Design review of the part built by this model. Coordinates are the model's own, in mm. Face numbers are marked on the shaded views. A direction names the side the tool comes from. Round coordinates to 2 decimals unless told otherwise and drop trailing zeros. Write each loop counter-clockwise with the first axis right and the second up, starting at its lowest first coordinate (ties: lowest second). Pieces come first, ordered by that corner, then holes. Notation, with made-up numbers: (21, 9.5) -> (45, 9.5) arc R21 cw to (45, 35.5) -> close; hole circle Ø11 at (-18, 38). An arc over 180 degrees is marked (long way). One line per question, with ' | ' between items. Start each with the question number.
1) Insertion check: pin 1 Ø0.9 at (x, y) = (-105.5, -7.5) entering from -Z; pin 2 Ø5 at (x, y) = (-97.5, 8.5) entering from +Z. Each pin has a flat end and moves straight along its axis. Give the tip position at first contact, or say it passes through.
2) Consider section A-A (z = 14.5). Give the boundary of the cut face in (x, y).
3) For the marked faces 1 and 2, list the 3-axis set-ups (+Z, -Z, +X, -X, +Y, -Y) from which the entire face can be reached by the end or side of a thin tool; tool diameter is ignored.
4) Consider section D-D (z = 6). Give the boundary of the cut face in (x, y), then the cut area to 3 significant figures.
5) Mouldability with a two-part tool opening along X and no side actions: class the marked faces 3, 4, 5 and 6 as +X half, -X half, draft (parallel to the pull), parting line (faces both ways), or undercut.
6) Consider section B-B (x = -92). Give the boundary of the cut face in (y, z), then the cut area to 3 significant figures.
7) For probe 1 along X at (y, z) = (1, 13.75); probe 2 along Y at (x, z) = (-91, 10.5); probe 3 along Z at (x, y) = (-87, -3.5), list the stretches that pass through material, from the lowest coordinate up.
8) Consider section C-C (y = 3). Give the boundary of the cut face in (x, z).
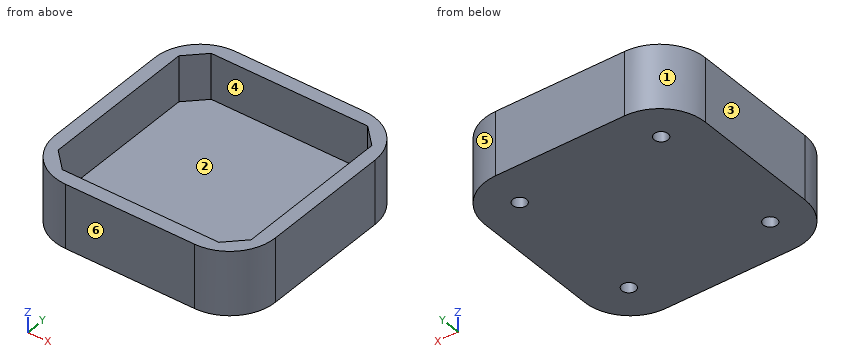
```python
from build123d import *

# Parameters (mm, degrees)
SKETCH1_W           = 48.3
SKETCH1_H           = 48.3
BOSS_EXTRUDE1_DEPTH = 10
SKETCH1_3_W         = 48.3
SKETCH1_3_H         = 48.3
SKETCH1_3_R         = 3.6
SKETCH1_3_R_2       = 6.5
BOSS_EXTRUDE2_DEPTH = 4
SKETCH2_R           = 1.5
CUT_EXTRUDE1_DEPTH  = 3.5
FILLET1_R           = 10


with BuildPart() as part:
    # Sketch1 → Boss-Extrude1 (new body)
    with BuildSketch(Plane(origin=(0, 0, 7.613932461), x_dir=(-1, 0, 0), z_dir=(0, 0, -1))):
        with Locations((89.733633233, 8.444815184)):
            Rectangle(SKETCH1_W, SKETCH1_H)
        Polygon((72.583633233, 29.594815184), (68.583633233, 25.594815184), (68.583633233, -8.705184816), (72.583633233, -12.705184816), (106.883633233, -12.705184816), (110.883633233, -8.705184816), (110.883633233, 25.594815184), (106.883633233, 29.594815184), align=None, mode=Mode.SUBTRACT)
    extrude(amount=-BOSS_EXTRUDE1_DEPTH)

    # Sketch1_3 → Boss-Extrude2 (add)
    with BuildSketch(Plane(origin=(0, 0, 7.613932461), x_dir=(-1, 0, 0), z_dir=(0, 0, -1))):
        with Locations((89.733633233, 8.444815184)):
            Rectangle(SKETCH1_3_W, SKETCH1_3_H)
        Polygon((72.583633233, 29.594815184), (68.583633233, 25.594815184), (68.583633233, -8.705184816), (72.583633233, -12.705184816), (106.883633233, -12.705184816), (110.883633233, -8.705184816), (110.883633233, 25.594815184), (106.883633233, 29.594815184), align=None, mode=Mode.SUBTRACT)
        Polygon((106.883633233, 29.594815184), (72.583633233, 29.594815184), (68.583633233, 25.594815184), (68.583633233, -8.705184816), (72.583633233, -12.705184816), (106.883633233, -12.705184816), (110.883633233, -8.705184816), (110.883633233, 25.594815184), align=None)
        Polygon((106.46941967, -11.705184816), (109.883633233, -8.290971253), (109.883633233, 25.180601622), (106.46941967, 28.594815184), (72.997846795, 28.594815184), (69.583633233, 25.180601622), (69.583633233, -8.290971253), (72.997846795, -11.705184816), align=None, mode=Mode.SUBTRACT)
        Polygon((72.997846795, -11.705184816), (106.46941967, -11.705184816), (109.883633233, -8.290971253), (109.883633233, 25.180601622), (106.46941967, 28.594815184), (72.997846795, 28.594815184), (69.583633233, 25.180601622), (69.583633233, -8.290971253), align=None)
        with Locations((105.233633233, -7.055184816)):
            Circle(SKETCH1_3_R, mode=Mode.SUBTRACT)
        with Locations((74.233633233, 23.944815184)):
            Circle(SKETCH1_3_R, mode=Mode.SUBTRACT)
        with Locations((89.733633233, 8.444815184)):
            Circle(SKETCH1_3_R_2, mode=Mode.SUBTRACT)
        with Locations((105.233633233, 23.944815184)):
            Circle(SKETCH1_3_R, mode=Mode.SUBTRACT)
        with Locations((74.233633233, -7.055184816)):
            Circle(SKETCH1_3_R, mode=Mode.SUBTRACT)
        with Locations((105.233633233, 23.944815184)):
            Circle(SKETCH1_3_R)
        with Locations((89.733633233, 8.444815184)):
            Circle(SKETCH1_3_R_2)
        with Locations((105.233633233, -7.055184816)):
            Circle(SKETCH1_3_R)
        with Locations((74.233633233, -7.055184816)):
            Circle(SKETCH1_3_R)
        with Locations((74.233633233, 23.944815184)):
            Circle(SKETCH1_3_R)
    extrude(amount=BOSS_EXTRUDE2_DEPTH)

    # Sketch2 → Cut-Extrude1 (cut)
    with BuildSketch(Plane(origin=(0, 0, 3.613932461), x_dir=(-1, 0, 0), z_dir=(0, 0, -1))):
        with Locations((105.233633233, 23.944815184)):
            Circle(SKETCH2_R)
        with Locations((105.233633233, -7.055184816)):
            Circle(SKETCH2_R)
        with Locations((74.233633233, -7.055184816)):
            Circle(SKETCH2_R)
        with Locations((74.233633233, 23.944815184)):
            Circle(SKETCH2_R)
    extrude(amount=-CUT_EXTRUDE1_DEPTH, mode=Mode.SUBTRACT)

    # Fillet1
    fillet1_edges = [part.edges().sort_by_distance(p)[0] for p in [
        (-65.583633233, 32.594815184, 10.613932461),
        (-113.883633233, 32.594815184, 10.613932461),
        (-113.883633233, -15.705184816, 10.613932461),
        (-65.583633233, -15.705184816, 10.613932461),
    ]]
    fillet(fillet1_edges, radius=FILLET1_R)


solid = part.part
```
From the geometry:
1) pin 1: stops at z = 7.11 | pin 2: stops at z = 7.61
2) outline: (-113.88, -5.71) arc R10 ccw to (-103.88, -15.71) -> (-75.58, -15.71) arc R10 ccw to (-65.58, -5.71) -> (-65.58, 22.59) arc R10 ccw to (-75.58, 32.59) -> (-103.88, 32.59) arc R10 ccw to (-113.88, 22.59) -> close; hole (-110.88, -8.71) -> (-106.88, -12.71) -> (-72.58, -12.71) -> (-68.58, -8.71) -> (-68.58, 25.59) -> (-72.58, 29.59) -> (-106.88, 29.59) -> (-110.88, 25.59) -> close
3) face 1: +Z, -Z, -X, +Y | face 2: +Z
4) outline: (-113.88, -5.71) arc R10 ccw to (-103.88, -15.71) -> (-75.58, -15.71) arc R10 ccw to (-65.58, -5.71) -> (-65.58, 22.59) arc R10 ccw to (-75.58, 32.59) -> (-103.88, 32.59) arc R10 ccw to (-113.88, 22.59) -> close; hole circle Ø3 at (-105.23, -7.06); hole circle Ø3 at (-105.23, 23.94); hole circle Ø3 at (-74.23, -7.06); hole circle Ø3 at (-74.23, 23.94) | area: 2,220 mm2
5) face 3: -X half | face 4: undercut | face 5: +X half | face 6: draft
6) outline: (-15.71, 3.61) -> (32.59, 3.61) -> (32.59, 17.61) -> (29.59, 17.61) -> (29.59, 7.61) -> (-12.71, 7.61) -> (-12.71, 17.61) -> (-15.71, 17.61) -> close | area: 253 mm2
7) probe 1: x = -113.88 to -110.88, -68.58 to -65.58 | probe 2: y = -15.71 to -12.71, 29.59 to 32.59 | probe 3: z = 3.61 to 7.61
8) outline: (-113.88, 3.61) -> (-65.58, 3.61) -> (-65.58, 17.61) -> (-68.58, 17.61) -> (-68.58, 7.61) -> (-110.88, 7.61) -> (-110.88, 17.61) -> (-113.88, 17.61) -> close
